For this review, use the dimensioned drawing (mm, ordinates from the lowest corner) and the shaded views. Coordinates: 2 decimals unless noted, no trailing zeros. Loops run counter-clockwise (first coordinate to the right, second up) from the corner with the lowest first, then second, coordinate; pieces in that order, holes last. Notation, with made-up numbers: M 31.25,43 L 63.25,43 A28 ccw 63.25,61 Z; hole C -19,71 d8. An arc over 180 degrees is marked long. One line per item, written item: value.
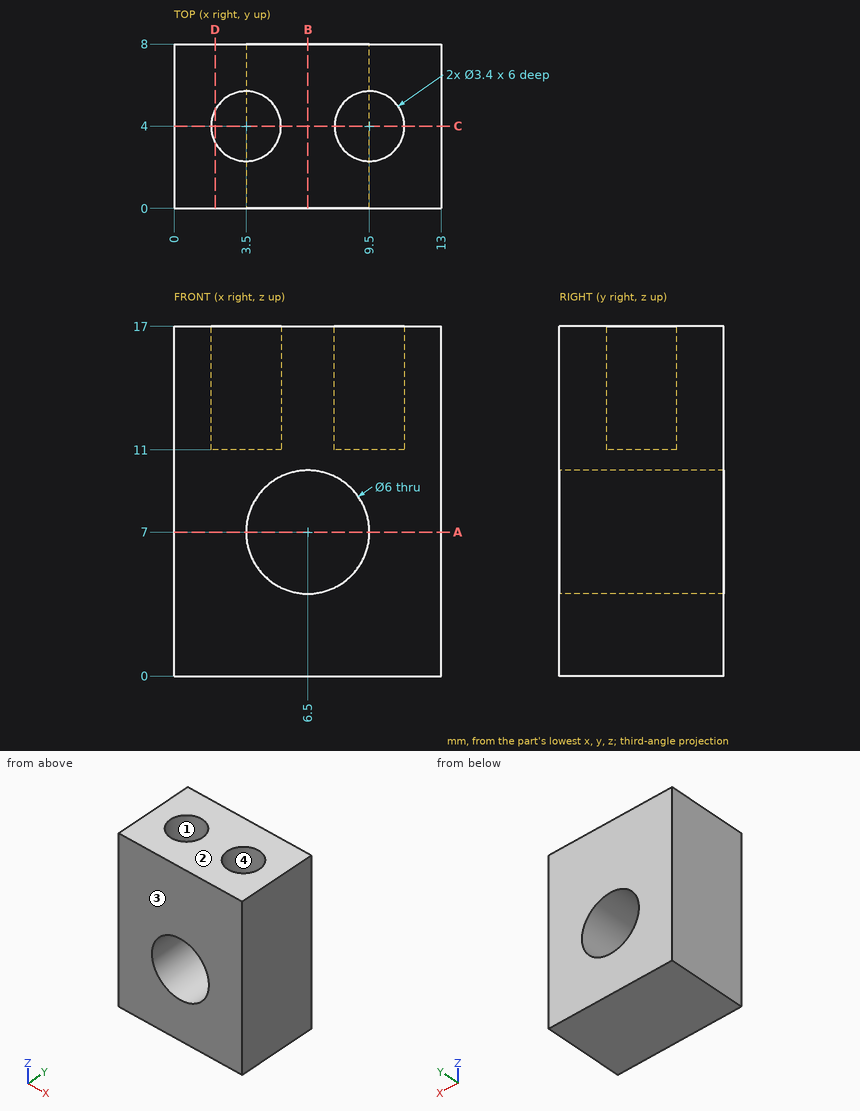
(1) We need section D-D on x = 2. State the section outline as (y, z) points, then the cut area to 3 significant figures.
Reply:
outline: M 0,0 L 8,0 L 8,17 L 4.8,17 L 4.8,11 L 3.2,11 L 3.2,17 L 0,17 Z
area: 126 mm2
(2) To check wall thickness, follow line 1 along Y through (x, z) = (9.5, 14.8); line 2 along Z through (x, y) = (6.5, 2.5); line 3 along X through (y, z) = (4, 6.75). State the ranges of each line that lie inside material, in increasing order. Write a range as [from, to].
Reply:
line 1: y = [0, 2.3], [5.7, 8]
line 2: z = [0, 4], [10, 17]
line 3: x = [0, 3.51], [9.49, 13]
(3) Insertion check: pin 1 (2.5 mm diameter, centred on x = 3.5, y = 4, fed in from +Z). The pin has a flat end and moves straight along its axis. Give the tip position at first contact, or say it passes through.
Reply:
pin 1: stops at z = 11
(4) We need section B-B on x = 6.5. State the section outline as (y, z) points.
Reply:
outline: M 0,0 L 8,0 L 8,4 L 0,4 Z; M 0,10 L 8,10 L 8,17 L 0,17 Z
(5) Mouldability with a two-part tool opening along Y and no side actions: class the marked faces 1, 2, 3 and 4 as released by +Y, released by -Y, zero draft, split by the parting line, or undercut.
Reply:
face 1: undercut
face 2: zero draft
face 3: released by -Y
face 4: undercut
(6) We need section C-C on y = 4. State the section outline as (x, z) points.
Reply:
outline: M 0,0 L 13,0 L 13,17 L 11.2,17 L 11.2,11 L 7.8,11 L 7.8,17 L 5.2,17 L 5.2,11 L 1.8,11 L 1.8,17 L 0,17 Z; hole C 6.5,7 d6
(7) We need section A-A on z = 7. State the section outline as (x, y) points, then the cut area to 3 significant figures.
Reply:
outline: M 0,0 L 3.5,0 L 3.5,8 L 0,8 Z; M 9.5,0 L 13,0 L 13,8 L 9.5,8 Z
area: 56.0 mm2
